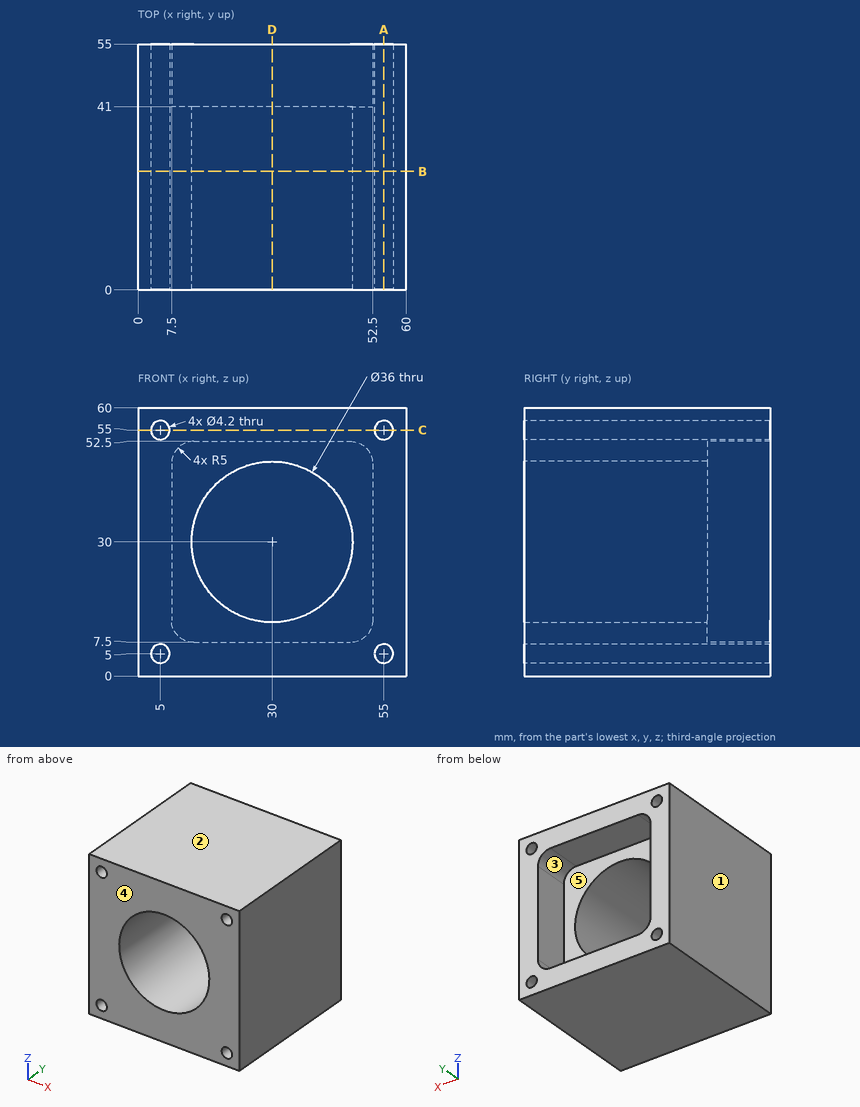
Source: three-view drawing plus pictorial views. Frame: mm from the lowest corner of the part. A direction names the side the tool comes from. Round coordinates to 2 decimals unless told otherwise and drop trailing zeros. Write each loop counter-clockwise with the first axis right and the second up, starting at its lowest first coordinate (ties: lowest second). Pieces come first, ordered by that corner, then holes. Notation, with made-up numbers: M 86.5,27.5 L 121.5,27.5 A21 ccw 121.5,65.5 Z; hole C -6,-31 d5. An arc over 180 degrees is marked long. One line per item, written item: value. Start each with the question number.
Item 1: Mould query, pull axis Z, two halves, no side actions, for the marked faces 1, 2 and 3. Classes: pulls with the +Z half, pulls with the -Z half, needs draft (parallel to the pull), parting line crosses it, or undercut.
Item 2: Set-up query: the marked faces 4 and 5. Return all of +Z, -Z, +X, -X, +Y, -Y with unobstructed straight access to the full face (end or side cutting, diameter ignored); none if empty.
Item 3: Section query D-D (x = 30). Return the cut outline in (y, z), plus the area to 3 significant figures.
Item 4: Section query A-A (x = 55). Return the cut outline in (y, z).
Item 5: Ray query, L1, parallel to X at y = 28, z = 5; L2, parallel to X at y = 48, z = 24. Return the intervals inside material, ascending. Write a range as from..to.
Item 6: Section query C-C (z = 55). Return the cut outline in (x, y), plus the area to 3 significant figures.
Item 7: Section query B-B (y = 26.5). Return the cut outline in (x, z).
Item 8: Pin query (flat end, axial travel): pin 1 (13.5 mm diameter, centred on x = 38.5, z = 21, fed in from +Y); pin 2 (4 mm diameter, centred on x = 5, z = 55, fed in from +Y). Return the tip coordinate at first contact, or that it passes through.
Result set:
1. face 1: needs draft
1. face 2: pulls with the +Z half
1. face 3: undercut
2. face 4: +Z, -Z, +X, -X, -Y
2. face 5: +Y
3. outline: M 0,0 L 55,0 L 55,7.5 L 41,7.5 L 41,12 L 0,12 Z; M 0,48 L 41,48 L 41,52.5 L 55,52.5 L 55,60 L 0,60 Z
3. area: 1,190 mm²
4. outline: M 0,0 L 55,0 L 55,2.9 L 0,2.9 Z; M 0,7.1 L 55,7.1 L 55,52.9 L 0,52.9 Z; M 0,57.1 L 55,57.1 L 55,60 L 0,60 Z
5. L1: x = 0..2.9, 7.1..52.9, 57.1..60
5. L2: x = 0..7.5, 52.5..60
6. outline: M 0,0 L 2.9,0 L 2.9,55 L 0,55 Z; M 7.1,0 L 52.9,0 L 52.9,55 L 7.1,55 Z; M 57.1,0 L 60,0 L 60,55 L 57.1,55 Z
6. area: 2,840 mm²
7. outline: M 0,0 L 60,0 L 60,60 L 0,60 Z; hole C 5,5 d4.2; hole C 5,55 d4.2; hole C 30,30 d36; hole C 55,5 d4.2; hole C 55,55 d4.2
8. pin 1: stops at y = 41
8. pin 2: passes through
